```python
from build123d import *

# Parameters (mm, degrees)
BOSS_EXTRUDE1_DEPTH = 15
SKETCH3_W           = 104.423940592
SKETCH3_H           = 121.358720552
CUT_EXTRUDE1_DEPTH  = 12
CUT_EXTRUDE2_DEPTH  = 3
CUT_EXTRUDE3_DEPTH  = 3
SKETCH6_R           = 18.828058828
SKETCH6_R_2         = 9.739436554
CUT_EXTRUDE4_DEPTH  = 5


with BuildPart() as part:
    # Sketch1 → Boss-Extrude1 (new body)
    with BuildSketch(Plane.XY):
        with BuildLine():
            Line((5, 0), (75, 0))
            ThreePointArc((75, 0), (78.535533906, 1.464466094), (80, 5))
            Line((80, 5), (80, 96.346))
            ThreePointArc((80, 96.346), (78.535533906, 99.881533906), (75, 101.346))
            Line((75, 101.346), (5, 101.346))
            ThreePointArc((5, 101.346), (1.464466094, 99.881533906), (0, 96.346))
            Line((0, 96.346), (0, 5))
            ThreePointArc((0, 5), (1.464466094, 1.464466094), (5, 0))
        make_face()
    extrude(amount=BOSS_EXTRUDE1_DEPTH)

    # Sketch3 → Cut-Extrude1 (cut)
    with BuildSketch(Plane.XY.offset(15)):
        with Locations((40, 50.673)):
            Rectangle(SKETCH3_W, SKETCH3_H)
        with BuildLine():
            Line((13.037037944, 4.371762639), (66.962962056, 4.371762639))
            ThreePointArc((66.962962056, 4.371762639), (74.034029868, 7.300694827), (76.962962056, 14.371762639))
            Line((76.962962056, 14.371762639), (76.962962056, 86.974237361))
            ThreePointArc((76.962962056, 86.974237361), (74.034029868, 94.045305173), (66.962962056, 96.974237361))
            Line((66.962962056, 96.974237361), (13.037037944, 96.974237361))
            ThreePointArc((13.037037944, 96.974237361), (5.965970132, 94.045305173), (3.037037944, 86.974237361))
            Line((3.037037944, 86.974237361), (3.037037944, 14.371762639))
            ThreePointArc((3.037037944, 14.371762639), (5.965970132, 7.300694827), (13.037037944, 4.371762639))
        make_face(mode=Mode.SUBTRACT)
    extrude(amount=-CUT_EXTRUDE1_DEPTH, mode=Mode.SUBTRACT)

    # Sketch4 → Cut-Extrude2 (cut)
    with BuildSketch(Plane.XY.offset(15)):
        with BuildLine():
            Line((36, 50.673), (3.037037944, 50.673))
            Line((3.037037944, 50.673), (3.037037944, 113.13523252))
            Line((3.037037944, 113.13523252), (76.962962056, 113.13523252))
            Line((76.962962056, 113.13523252), (76.962962056, 66.159087484))
            Line((76.962962056, 66.159087484), (44, 66.159087484))
            ThreePointArc((44, 66.159087484), (41.171572875, 64.987514609), (40, 62.159087484))
            Line((40, 62.159087484), (40, 54.673))
            ThreePointArc((40, 54.673), (38.828427125, 51.844572875), (36, 50.673))
        make_face()
    extrude(amount=-CUT_EXTRUDE2_DEPTH, mode=Mode.SUBTRACT)

    # Sketch5 → Cut-Extrude3 (cut)
    with BuildSketch(Plane.XY.offset(15)):
        with BuildLine():
            Line((83.710638267, 26.274744542), (68.481884822, 26.274744542))
            ThreePointArc((68.481884822, 26.274744542), (57.451328272, 37.305301092), (68.481884822, 48.335857641))
            Line((68.481884822, 48.335857641), (83.710638267, 48.335857641))
            ThreePointArc((83.710638267, 48.335857641), (94.741194817, 37.305301092), (83.710638267, 26.274744542))
        make_face()
    extrude(amount=-CUT_EXTRUDE3_DEPTH, mode=Mode.SUBTRACT)

    # Sketch6 → Cut-Extrude4 (cut)
    with BuildSketch(Plane.XY.offset(15)):
        with Locations((40, 4.371762639)):
            Circle(SKETCH6_R)
        with Locations((40, 4.371762639)):
            Circle(SKETCH6_R_2, mode=Mode.SUBTRACT)
    extrude(amount=-CUT_EXTRUDE4_DEPTH, mode=Mode.SUBTRACT)


solid = part.part
```
Can you work these out from the model? Positions are in its coordinate system, mm. A direction names the side the tool comes from. Coordinates: 2 decimals unless noted, no trailing zeros. Loops run counter-clockwise (first coordinate to the right, second up) from the corner with the lowest first, then second, coordinate; pieces in that order, holes last. Notation, with made-up numbers: (3.5, -13) -> (50.5, -13) arc R13 cw to (50.5, 5) -> close; hole circle Ø7 at (23, 73.5). An arc over 180 degrees is marked (long way). Put each result on its own line as item: value. Start each with the question number.
Q1. For faces 1 (the face through (76.963, 50, 9)), 2 (the face through (3.037, 51, 9)), 3 (the face through (40, 4.372, 8)), 4 (the face through (73, 26.275, 14)), 5 (the face through (73.956, 7.223, 9.084)), which set-ups out of +Z, -Z, +X, -X, +Y, -Y let a thin tool reach every point of the face, with its end or its side?
Q2. I want a section at A-A (y = 85). Write out the boundary of the cut face in (x, z), plus the area to 3 significant figures.
Q3. I want a section at B-B (x = 16.5). Write out the boundary of the cut face in (y, z).
Q4. I'm going to push flat-ended pins straight in: P1, Ø3, axis at y = 37.5, z = 8.5, coming from the +X side; P2, Ø1.5, axis at x = 22, z = 7.5, coming from the +Y side; P3, Ø2.5, axis at x = 74, z = 14, coming from the -Y side. Where does each tip first touch, or does it pass through?
Q5. I want a section at C-C (z = 8). Write out the boundary of the cut face in (x, y).
Q6. Thinking about a two-plate mould opening in Y: for faces 6 (the face through (38.859, 51.876, 13.521)), 7 (the face through (0, 51, 1)), 8 (the face through (73, 48.336, 14)), which applies, pulls with the +Y half, pulls with the -Y half, needs draft (parallel to the pull), parting line crosses it, or undercut?
Q7. If I drill on line 1 (Z direction, x = 22, y = 84); line 2 (X direction, y = 61.5, z = 6); line 3 (Y direction, x = 63.5, z = 11.25), over which ranges is the centre line in solid material (lowest first)? Write a range as [from, to].
Q8. I want a section at D-D (x = 26.5). Write out the boundary of the cut face in (y, z).
Taken from the geometry:
1. face 1: +Z, +X, +Y, -Y
1. face 2: +Z, -X, +Y, -Y
1. face 3: +Z, +X, -X, -Y
1. face 4: +Z, +X
1. face 5: +Z, +X, -Y
2. outline: (0, 0) -> (80, 0) -> (80, 3) -> (76.96, 3) -> (76.96, 12) -> (3.04, 12) -> (3.04, 3) -> (0, 3) -> close
2. area: 905 mm2
3. outline: (0, 0) -> (101.35, 0) -> (101.35, 3) -> (96.97, 3) -> (96.97, 12) -> (50.67, 12) -> (50.67, 15) -> (4.37, 15) -> (4.37, 3) -> (0, 3) -> close
4. P1: stops at x = 76.96
4. P2: stops at y = 96.97
4. P3: stops at y = 6.22
5. outline: (3.04, 14.37) arc R10 ccw to (13.04, 4.37) -> (66.96, 4.37) arc R10 ccw to (76.96, 14.37) -> (76.96, 86.97) arc R10 ccw to (66.96, 96.97) -> (13.04, 96.97) arc R10 ccw to (3.04, 86.97) -> close
6. face 6: pulls with the +Y half
6. face 7: needs draft
6. face 8: undercut
7. line 1: z = [0, 12]
7. line 2: x = [3.04, 76.96]
7. line 3: y = [4.37, 96.97]
8. outline: (0, 0) -> (101.35, 0) -> (101.35, 3) -> (96.97, 3) -> (96.97, 12) -> (50.67, 12) -> (50.67, 15) -> (17.5, 15) -> (17.5, 10) -> (4.37, 10) -> (4.37, 3) -> (0, 3) -> close
